Source: three-view drawing plus pictorial views. Frame: mm from the lowest corner of the part. Round coordinates to 2 decimals unless told otherwise and drop trailing zeros. Loops run counter-clockwise (first coordinate to the right, second up) from the corner with the lowest first, then second, coordinate; pieces in that order, holes last. Notation, with made-up numbers: M 83,7.25 L 134,7.25 A34 cw 134,42.25 Z; hole C 45.25,-27.75 d1. An arc over 180 degrees is marked long. Return JSON: item names as keys, results as strings. Group by question number.
1) Material intervals for line 1 (Z direction, x = 34.5, y = 14); line 2 (Y direction, x = 20, z = 3.7); line 3 (Y direction, x = 22, z = 1.75), sorted ascending. Write a range as from..to.
2) Section A-A (y = 20). Output: boundary loops of the cut face in (x, z), plus the area to 3 significant figures.
3) Mould query, pull axis X, two halves, no side actions, for the marked faces 1 and 2. Classes: +X half, -X half, draft (parallel to the pull), parting line (faces both ways), or undercut.
4) Contact query for flat-ended pins moving along their axis: P1, Ø2, axis at y = 19.5, z = 7, coming from the -X side; P2, Ø6, axis at x = 33.5, y = 33, coming from the -Z side; P3, Ø6, axis at y = 24.5, z = 5, coming from the +X side; P4, Ø16, axis at x = 20, y = 20, coming from the +Z side. Output: stop coordinate, or through.
5) Section D-D (z = 4). Output: boundary loops of the cut face in (x, y).
6) Section C-C (z = 1.5). Output: boundary loops of the cut face in (x, y).
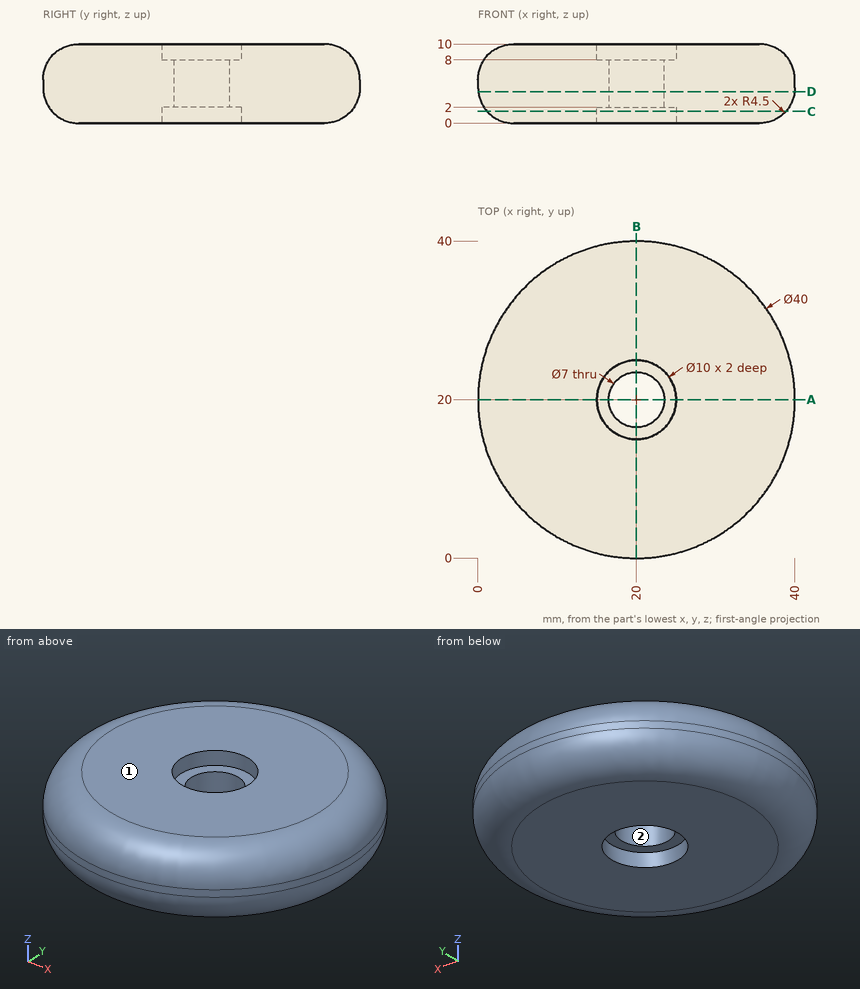
Returned:
{
 "1": {"line 1": "z = 0..10", "line 2": "y = 0.07..16.5, 23.5..39.93", "line 3": "y = 1.04..15.42, 24.58..38.96"},
 "2": {"outline": "M 0,4.5 A4.5 ccw 4.5,0 L 15,0 L 15,2 L 16.5,2 L 16.5,8 L 15,8 L 15,10 L 4.5,10 A4.5 ccw 0,5.5 Z; M 23.5,2 L 25,2 L 25,0 L 35.5,0 A4.5 ccw 40,4.5 L 40,5.5 A4.5 ccw 35.5,10 L 25,10 L 25,8 L 23.5,8 Z", "area": "301 mm^2"},
 "3": {"face 1": "draft", "face 2": "undercut"},
 "4": {"P1": "stops at x = 0.03", "P2": "stops at z = 0.01", "P3": "stops at x = 39.94", "P4": "stops at z = 10"},
 "5": {"outline": "C 20,20 d39.94; hole C 20,20 d7"},
 "6": {"outline": "C 20,20 d37.71; hole C 20,20 d10"}
}
